Design review of the part built by this model. Coordinates are the model's own, in mm. A direction names the side the tool comes from. Coordinates: 2 decimals unless noted, no trailing zeros. Order: outer loops, then holes, each group sorted by start corner. A loop starts at its lowest first (then second) coordinate and runs counter-clockwise, first axis right, second up. Notation, with made-up numbers: M 74.25,-14.75 L 112.25,-14.75 A12 ccw 112.25,-10.75 Z; hole C 40,6 d3. An arc over 180 degrees is marked long. Answer in a Markdown table with one row per item.
Autodesk Inventor part; units mm, degrees
ref_plane "YZ Plane" through (0, 0, 0) normal (1, 0, 0) x (0, 1, 0)
ref_plane "XZ Plane" through (0, 0, 0) normal (0, 1, 0) x (-1, 0, 0)
ref_plane "XY Plane" through (0, 0, 0) normal (0, 0, 1) x (1, 0, 0)
sketch "Sketch1" plane through (0, 0, 0) normal (0, 0, 1) x (1, 0, 0)
  line L0 (-10, 0) -> (0, 0)
  line L1 (-10, 0) -> (-10, 20)
  line L2 (-10, 20) -> (-7.5, 20)
  line L3 (-4.5, 20) -> (-1.5, 20)
  line L4 (-7.5, 20) -> (-6, 18.5)
  line L5 (-6, 18.5) -> (-4.5, 20)
  line L6 (-1.5, 20) -> (0, 18.5)
  line L7 (0, 18.5) -> (0, 0) construction
  line L8 (10, 0) -> (0, 0)
  line L9 (10, 0) -> (10, 20)
  line L10 (10, 20) -> (7.5, 20)
  line L11 (4.5, 20) -> (1.5, 20)
  line L12 (7.5, 20) -> (6, 18.5)
  line L13 (6, 18.5) -> (4.5, 20)
  line L14 (1.5, 20) -> (0, 18.5)
  circle A0 centre (0, 10) radius 3
  dimension "d0" = 6
  dimension "d1" = 20
  dimension "d2" = 20
  dimension "d3" = 1.5
  dimension "d4" = 6
  dimension "d5" = 10
extrude "Extrusion1" add sketch "Sketch1" along normal mid plane 19.6
sketch "Sketch2" plane through (10, 0, 9.8) normal (1, 0, 0) x (0, 0, -1)
  line L0 (19.6, 20) -> (0, 20)
  line L1 (9.8, 20) -> (9.8, 0) construction
  line L2 (0, 13) -> (19.6, 13)
  line L3 (2.3, 20) -> (3.8, 18.5)
  line L4 (3.8, 18.5) -> (5.3, 20)
  line L5 (19.6, 20) -> (0, 20)
  line L6 (8.3, 20) -> (9.8, 18.5)
  line L7 (17.3, 20) -> (15.8, 18.5)
  line L8 (15.8, 18.5) -> (14.3, 20)
  line L9 (11.3, 20) -> (9.8, 18.5)
  dimension "d8" = 1.5
  dimension "d9" = 6
extrude "Extrusion2" cut sketch "Sketch2" against normal through all
chamfer "Chamfer1" distance 0.5 angle 45 1 edges at (-3, 10, 9.8)
properties part number "Foot" material "Steel"
(1) Draft analysis for pull direction Z (two halves, no side actions). For faces 4 (the flat face through (6.8, 19.3, 8.3)), 5 (the flat face through (3, 19.1, -6.6)), state which applies: pulls with the +Z half, pulls with the -Z half, needs draft (parallel to the pull), parting line crosses it, or undercut.
Return value:
| item | result |
|---|---|
| face 4 | needs draft |
| face 5 | undercut |
(2) Add section C-C, the plane x = 4. Give the boundary of the cut face in (y, z), and give its area (3 significant figures).
Return value:
| item | result |
|---|---|
| outline | M 0,-9.8 L 20,-9.8 L 20,-7.5 L 18.5,-6 L 20,-4.5 L 20,-1.5 L 18.5,0 L 20,1.5 L 20,4.5 L 18.5,6 L 20,7.5 L 20,9.8 L 0,9.8 Z |
| area | 385 mm2 |
(3) Insertion check: pin 1 Ø5 at (x, z) = (0.5, -4.5) entering from -Y. The pin has a flat end and moves straight along its axis. Give the tip position at first contact, or say it passes through.
Return value:
| item | result |
|---|---|
| pin 1 | stops at y = 0 |
(4) For line 1 along X through (y, z) = (12.5, 0); line 2 along Y through (x, z) = (0.25, 7); line 3 along Y through (x, z) = (-6.25, -7.25), list the stretches that pass through material, from the lowest coordinate up. Write a range as from..to.
Return value:
| item | result |
|---|---|
| line 1 | x = -10..-1.66, 1.66..10 |
| line 2 | y = 0..7.01, 12.99..18.75 |
| line 3 | y = 0..18.75 |
(5) For faces 1 (the flat face through (0.6, 19.1, -3)), 2 (the flat face through (8.5, 19.2, -5.3)), 3 (the flat face through (-3, 20, -3)), list the 3-axis set-ups (+Z, -Z, +X, -X, +Y, -Y) from which the entire face can be reached by the end or side of a thin tool; tool diameter is ignored.
Return value:
| item | result |
|---|---|
| face 1 | +Z, -Z, +Y |
| face 2 | +X, -X, +Y |
| face 3 | +Z, -Z, +X, -X, +Y |
(6) Add section D-D, the plane z = 2. Give the boundary of the cut face in (x, y).
Return value:
| item | result |
|---|---|
| outline | M -10,0 L 10,0 L 10,20 L 7.5,20 L 6,18.5 L 4.5,20 L 1.5,20 L 0,18.5 L -1.5,20 L -4.5,20 L -6,18.5 L -7.5,20 L -10,20 Z; hole C 0,10 d6 |
(7) Add section A-A, the plane z = -5. Give the boundary of the cut face in (x, y), and give its area (3 significant figures).
Return value:
| item | result |
|---|---|
| outline | M -10,0 L 10,0 L 10,19.5 L 7,19.5 L 6,18.5 L 5,19.5 L 1,19.5 L 0,18.5 L -1,19.5 L -5,19.5 L -6,18.5 L -7,19.5 L -10,19.5 Z; hole C 0,10 d6 |
| area | 359 mm2 |
(8) Add section B-B, the plane y = 10. Give the boundary of the cut face in (x, z), and give its area (3 significant figures).
Return value:
| item | result |
|---|---|
| outline | M -10,-9.8 L -3,-9.8 L -3,9.3 L -3.5,9.8 L -10,9.8 Z; M 3,-9.8 L 10,-9.8 L 10,9.8 L 3.5,9.8 L 3,9.3 Z |
| area | 274 mm2 |
